```python
from build123d import *

# Parameters (mm, degrees)
SKETCH1_R                = 36.5
SKETCH1_R_2              = 35
BOSS_EXTRUDE1_DEPTH      = 20
BOSS_EXTRUDE2_DEPTH      = 120
BOSS_EXTRUDE2_DEPTH_BACK = 5
SKETCH3_R                = 38
SKETCH3_R_2              = 36.5
CHAMFER1_SIZE            = 2
SKETCH4_R                = 37.15
CUT_EXTRUDE1_DEPTH       = 120


with BuildPart() as part:
    # Sketch1 → Boss-Extrude1 (new body)
    with BuildSketch(Plane(origin=(0, 0, 0), x_dir=(1, 0, 0), z_dir=(0, 1, 0))):
        with Locations(Location((0, 0, 0), (0, 0, 270))):
            Circle(SKETCH1_R)
        with Locations(Location((0, 0, 0), (0, 0, 270))):
            Circle(SKETCH1_R_2, mode=Mode.SUBTRACT)
    extrude(amount=BOSS_EXTRUDE1_DEPTH)

    # Sketch2 → Revolve1 (revolve)
    with BuildSketch(Plane.XY, mode=Mode.PRIVATE) as revolve1_sk:
        with BuildLine():
            Line((-35, 20), (-36.5, 20))
            add(Edge.make_bspline(
                [(-36.5, 20), (-36.5, 20.938203754), (-36.489872815, 22.828803886), (-36.429914329, 26.496139533), (-36.282028405, 30.946908345), (-35.992678983, 36.053561075), (-35.464097096, 42.564076378), (-34.547626097, 50.148542942), (-33.076762757, 58.396561812), (-31.272577792, 65.822093819), (-28.472409657, 74.667565146), (-24.325017143, 83.822828988), (-18.603719652, 92.00577673), (-13.454241979, 96.674123666), (-9.254678436, 99.216783088), (-6.104208908, 100.550031186), (-3.516650787, 101.201383216), (-1.484729716, 101.45792619), (-0.497779404, 101.5), (0, 101.5)],
                knots=[0, 0, 0, 0, 0.015625, 0.03125, 0.0625, 0.09375, 0.125, 0.1875, 0.25, 0.3125, 0.375, 0.5, 0.625, 0.75, 0.8125, 0.875, 0.9375, 0.96875, 1, 1, 1, 1], degree=3))
            Line((0, 101.5), (0, 100))
            add(Edge.make_bspline(
                [(-35, 20), (-35, 80.332266649), (-14.376326679, 100), (0, 100)],
                knots=[0, 0, 0, 0, 1, 1, 1, 1], degree=3))
        make_face()
    revolve(revolve1_sk.sketch.rotate(Axis((0, 20, 0), (0, 1, 0)), 270), axis=Axis((0, 20, 0), (0, 1, 0)))

    # Sketch3 → Boss-Extrude2 (add, two sides: drawn at the far end of the back side and taken through both)
    with BuildSketch(Plane.XZ.offset(-BOSS_EXTRUDE2_DEPTH_BACK)):
        with Locations(Location((0, 0, 0), (0, 0, 270))):
            Circle(SKETCH3_R)
        with Locations(Location((0, 0, 0), (0, 0, 270))):
            Circle(SKETCH3_R_2, mode=Mode.SUBTRACT)
    extrude(amount=BOSS_EXTRUDE2_DEPTH + BOSS_EXTRUDE2_DEPTH_BACK)

    # Chamfer1
    # the kernel refuses this chamfer: 2 mm, written as the material it takes off along each edge
    with BuildSketch(Plane(origin=(0, 5, 0), x_dir=(0, 0, -1), z_dir=(-1, 0, 0))) as chamfer1_piece_1_section:
        Polygon((38 - CHAMFER1_SIZE, 0), (38, CHAMFER1_SIZE), (38, 0), align=None)
    chamfer1_piece_1 = revolve(axis=Axis((0, 5, 0), (0, -1, 0)), mode=Mode.PRIVATE)
    chamfer1_piece_1 = chamfer1_piece_1 - Plane(origin=(0, 3.777023611, 0), x_dir=(0, 0, 1), z_dir=(0, -1, 0)) * Cylinder(36.5, 153, mode=Mode.PRIVATE)
    add(chamfer1_piece_1, mode=Mode.SUBTRACT)

    # Sketch4 → Cut-Extrude1 (cut)
    with BuildSketch(Plane.XZ.offset(120)):
        with Locations(Location((0, 0, 0), (0, 0, 270))):
            Circle(SKETCH4_R)
    extrude(amount=-CUT_EXTRUDE1_DEPTH, mode=Mode.SUBTRACT)


solid = part.part
```
Source: CAD feature listing. Evaluate the final solid. Frame: model axes, mm. Round coordinates to 2 decimals unless told otherwise and drop trailing zeros. Loops run counter-clockwise (first coordinate to the right, second up) from the corner with the lowest first, then second, coordinate; pieces in that order, holes last.
1. Section query A-A on y = -77.5. Output: boundary loops of the cut face in (x, z), and give its area (3 significant figures).
2. Mould query, pull axis X, two halves, no side actions, for faces 1 (the cylindrical face through (-21, 10, -28)), 2 (the cylindrical face through (-23.122, -57.639, 30.156)), 3 (the cylindrical face through (11.159, -60.84, -35.434)), 4 (the flat face through (-36.4, -120, -8.3)). Classes: released by +X, released by -X, zero draft, split by the parting line, or undercut.
3. Ray query, L1, parallel to X at y = 6.75, z = 0; L2, parallel to X at y = -67, z = 0; L3, parallel to Z at x = 18, y = 74. Return the intervals inside material, ascending.
4. Contact query for flat-ended pins moving along their axis: pin 1 (12 mm diameter, centred on x = 25.5, z = -16.5, fed in from -Y); pin 2 (12 mm diameter, centred on x = -3, y = 61.5, fed in from +Z); pin 3 (6 mm diameter, centred on y = 62, z = 27.5, fed in from +X). Output: stop coordinate, or through.
Answers below:
1. outline: circle Ø76 at (0, 0); hole circle Ø74.3 at (0, 0)
1. area: 201 mm2
2. face 1: undercut
2. face 2: split by the parting line
2. face 3: undercut
2. face 4: zero draft
3. L1: x = -36.5 to -35, 35 to 36.5
3. L2: x = -38 to -37.15, 37.15 to 38
3. L3: z = -22.11 to -20, 20 to 22.11
4. pin 1: stops at y = 0
4. pin 2: stops at z = 33.5
4. pin 3: stops at x = 21.03
